Check sheet for the modelled part. Datum: model origin and axes. Units: mm. A direction names the side the tool comes from. Round coordinates to 2 decimals unless told otherwise and drop trailing zeros. Write each loop counter-clockwise with the first axis right and the second up, starting at its lowest first coordinate (ties: lowest second). Pieces come first, ordered by that corner, then holes.
Item 1: Cross-section at A-A on y = 22. Enter the section's corners in (x, z).
Item 2: Tool access check on faces 5 (the flat face through (5.5, 11, -0.2)), 6 (the cylindrical face through (-0.601, 28.092, 9.93)), 7 (the flat face through (0, 15, 0)), 8 (the flat face through (-9, 1, 0)). Record the directions out of +Z, -Z, +X, -X, +Y, -Y that give a thin tool (end or side, any length) a straight path to the whole face; none if there is none.
Item 3: Material ranges on line 1 (Z direction, x = 3, y = 30); line 2 (X direction, y = 30, z = -7.5); line 3 (Y direction, x = 0, z = 10.5), recorded low to high.
Item 4: Cross-section at B-B on x = 0. Enter the section's corners in (y, z).
Item 5: Cross-section at C-C on z = 0. Enter the section's corners in (x, y), plus the area to 3 significant figures.
Item 6: Release check for a two-part mould opening along X. For faces 1 (the flat face through (-5, 23, -7)), 2 (the cylindrical face through (-0.601, 28.092, -10.07)), 3 (the cylindrical face through (12.56, 0.51, 0.35)), 4 (the flat face through (5, 23, -7)) record: +X half, -X half, draft (parallel to the pull), parting line (faces both ways), or undercut.
Item 7: Cross-section at D-D on x = 11. Enter the section's corners in (y, z), plus the area to 3 significant figures.
Item 8: Go/stop test with flat-tipped pins: pin 1 Ø3 at (x, y) = (0, 30) entering from -Z; pin 2 Ø0.8 at (x, z) = (-5.5, 0.5) entering from +Y; pin 3 Ø5 at (x, z) = (11, 0) entering from -Y; pin 4 Ø5 at (x, z) = (10, 3) entering from +Y. Record where each tip stops, or that it passes through.
Autodesk Inventor part; units mm, degrees
ref_plane "YZ Plane" through (0, 0, 0) normal (1, 0, 0) x (0, 1, 0)
ref_plane "XZ Plane" through (0, 0, 0) normal (0, 1, 0) x (-1, 0, 0)
ref_plane "XY Plane" through (0, 0, 0) normal (0, 0, 1) x (1, 0, 0)
sketch "Náčrt1" plane through (0, 0, 0) normal (0, 0, 1) x (1, 0, 0)
  line L0 (-9.2032, 0) -> (20.2005, 0)
  line L1 (0, 42) -> (0, -7)
  line L2 (-5.0026, 0) -> (16, 0)
  line L3 (16, 0) -> (16, 1)
  line L4 (16, 1) -> (6, 1)
  line L5 (6, 1) -> (6, 11)
  line L6 (6, 11) -> (5, 11)
  line L7 (5, 11) -> (5, 35)
  line L8 (5, 35) -> (0, 35)
  line L9 (0, 35) -> (0, 0)
  line L10 (0, 0) -> (-5.0026, 0)
  line L11 (0, 0) -> (16, 0)
  point P0 (0, 0)
  point P1 (0, 35)
  point P2 (16, 0)
  dimension "d0" = 10
  dimension "d1" = 10
  dimension "d2" = 1
  dimension "d3" = 1
  dimension "d4" = 5
  dimension "d5" = 35
extrude "Vysunutí1" add sketch "Náčrt1" along normal mid plane 30
mirror "Zrcadlit1" about plane through (0, 35, 0) normal (-1, 0, 0) of "Vysunutí1"
sketch "Náčrt2" plane through (5, 11, 15) normal (1, 0, 0) x (0, 0, -1)
  line L0 (0, 24) -> (30, 24)
  line L1 (0, 0) -> (0, 24)
  line L2 (30, 0) -> (0, 0)
  line L3 (30, 24) -> (30, 0)
  line L4 (10, 24) -> (20, 24)
  line L5 (20, 24) -> (20, 4)
  line L6 (20, 4) -> (10, 4)
  line L7 (10, 4) -> (10, 24)
  line L8 (10, 24) -> (20, 24)
  point P0 (15, -11)
  point P1 (10, 0)
  point P2 (20, 0)
  dimension "d8" = 10
  dimension "d9" = 10
  dimension "d10" = 20
extrude "Vysunutí3" cut sketch "Náčrt2" against normal through all contours L0 L5 L6 L7
sketch "Náčrt3" plane through (0, 0, 15) normal (0, 0, 1) x (1, 0, 0)
  line L0 (5, 35) -> (-5, 35)
  line L1 (-5, 11) -> (-5, 35)
  line L2 (-6, 11) -> (-5, 11)
  line L3 (-6, 1) -> (-6, 11)
  line L4 (-16, 1) -> (-6, 1)
  line L5 (-16, 0) -> (-16, 1)
  line L6 (16, 0) -> (-16, 0)
  line L7 (16, 0) -> (16, 1)
  line L8 (16, 1) -> (6, 1)
  line L9 (6, 1) -> (6, 11)
  line L10 (6, 11) -> (5, 11)
  line L11 (5, 11) -> (5, 35)
  point P0 (0, 0)
  point P1 (0, 30)
  dimension "d15" = 5
  dimension "d16" = 5
hole "Díra1" at (0, 30, 15) direction (0, 0, -1) diameter 4 end through all
sketch "Náčrt4" plane through (16, 0, -15) normal (0, -1, 0) x (1, 0, 0)
  line L0 (-10, 0) -> (-10, 30)
  line L1 (0, 0) -> (0, 30)
  line L2 (0, 30) -> (-32, 30)
  line L3 (-32, 0) -> (-32, 30)
  line L4 (0, 0) -> (-32, 0)
  point P0 (-16, 15)
  point P1 (-5, 15)
  point P2 (-27, 15)
  dimension "d24" = 5
  dimension "d27" = 15
  dimension "d28" = 15
  dimension "d31" = 5
hole "Díra2" at (11, 0, 0) at (-11, 0, 0) direction (0, 1, 0) diameter 3.2 end through all
properties part number "y_bearing_holder"
Response values:
1. outline: (-5, -15) - (5, -15) - (5, -5) - (-5, -5) - close; (-5, 5) - (5, 5) - (5, 15) - (-5, 15) - close
2. face 5: +Z, -Z, +X, +Y
2. face 6: +Z, -Z
2. face 7: +X, -X, +Y
2. face 8: +Z, -Z, -X, +Y
3. line 1: z = -15 to -5, 5 to 15
3. line 2: x = -5 to -2, 2 to 5
3. line 3: y = 0 to 28, 32 to 35
4. outline: (0, -15) - (28, -15) - (28, -5) - (15, -5) - (15, 5) - (28, 5) - (28, 15) - (0, 15) - close; (32, -15) - (35, -15) - (35, -5) - (32, -5) - close; (32, 5) - (35, 5) - (35, 15) - (32, 15) - close
5. outline: (-16, 0) - (-12.6, 0) - (-12.6, 1) - (-16, 1) - close; (-9.4, 0) - (9.4, 0) - (9.4, 1) - (6, 1) - (6, 11) - (5, 11) - (5, 15) - (-5, 15) - (-5, 11) - (-6, 11) - (-6, 1) - (-9.4, 1) - close; (12.6, 0) - (16, 0) - (16, 1) - (12.6, 1) - close
5. area: 186 mm2
6. face 1: -X half
6. face 2: undercut
6. face 3: undercut
6. face 4: +X half
7. outline: (0, -15) - (1, -15) - (1, -1.6) - (0, -1.6) - close; (0, 1.6) - (1, 1.6) - (1, 15) - (0, 15) - close
7. area: 26.8 mm2
8. pin 1: passes through
8. pin 2: stops at y = 11
8. pin 3: stops at y = 0
8. pin 4: stops at y = 1
